Could you check a few things on this model? Use its own coordinates, in mm. Coordinates: 2 decimals unless noted, no trailing zeros. Write each loop counter-clockwise with the first axis right and the second up, starting at its lowest first coordinate (ties: lowest second). Pieces come first, ordered by that corner, then holes. Notation, with made-up numbers: (61, 27) - (117, 27) arc R29 ccw to (117, 51) - close; hole circle Ø11 at (22.25, 39.5). An arc over 180 degrees is marked (long way). Answer as a JSON object with one key per item and string values. Group by question number.
1) Will these pins go through, and if not, where does the flat tip stop? pin 1 Ø7.5 at (x, y) = (56, 6.5) entering from +Z; pin 2 Ø5.5 at (x, y) = (5, 5) entering from +Z.
2) If we section it at A-A (y = 5): Write out the boundary of the cut face in (x, z).
3) Please list where these lines run through material, in increasing order: line 1 along Y through (x, z) = (55, 0.55); line 2 along Y through (x, z) = (5, 1.9); line 3 along Y through (x, z) = (54, 3.4).
4) If we section it at D-D (z = 2.7): Write out the boundary of the cut face in (x, y).
5) If we section it at C-C (y = 55): Write out the boundary of the cut face in (x, z).
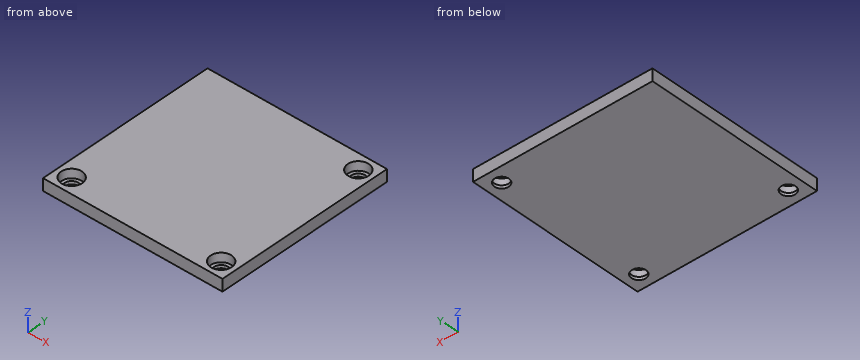
```python
from build123d import *

# Parameters (mm, degrees)
CYLINDER005_R     = 3.5
CYLINDER005_DEPTH = 3
CYLINDER004_R     = 2.4
CYLINDER004_DEPTH = 10
CYLINDER007_R     = 3.5
CYLINDER007_DEPTH = 3
CYLINDER006_R     = 2.4
CYLINDER006_DEPTH = 10
CYLINDER009_R     = 3.5
CYLINDER009_DEPTH = 3
CYLINDER008_R     = 2.4
CYLINDER008_DEPTH = 10
BOX001_W          = 60
BOX001_H          = 60
BOX001_DEPTH      = 4


with BuildPart() as cylinder005:
    # Cylinder005 → Cylinder005 (new body)
    with BuildSketch(Plane.XY.offset(1)):
        Circle(CYLINDER005_R)
    extrude(amount=CYLINDER005_DEPTH)


with BuildPart() as fusion004:
    # Cylinder004 → Cylinder004 (new body)
    with BuildSketch(Plane.XY):
        Circle(CYLINDER004_R)
    extrude(amount=CYLINDER004_DEPTH)

    # Fusion004: union Cylinder005
    add(cylinder005.part)


with BuildPart() as fusion004_1:
    # Fusion004 placement: moved
    add(fusion004.part.moved(Location((5, 5, 0))))


with BuildPart() as cylinder007:
    # Cylinder007 → Cylinder007 (new body)
    with BuildSketch(Plane.XY.offset(1)):
        Circle(CYLINDER007_R)
    extrude(amount=CYLINDER007_DEPTH)


with BuildPart() as fusion005:
    # Cylinder006 → Cylinder006 (new body)
    with BuildSketch(Plane.XY):
        Circle(CYLINDER006_R)
    extrude(amount=CYLINDER006_DEPTH)

    # Fusion005: union Cylinder007
    add(cylinder007.part)


with BuildPart() as fusion005_1:
    # Fusion005 placement: moved
    add(fusion005.part.moved(Location((55, 5, 0))))


with BuildPart() as cylinder009:
    # Cylinder009 → Cylinder009 (new body)
    with BuildSketch(Plane.XY.offset(1)):
        Circle(CYLINDER009_R)
    extrude(amount=CYLINDER009_DEPTH)


with BuildPart() as compound001:
    # Cylinder008 → Cylinder008 (new body)
    with BuildSketch(Plane.XY):
        Circle(CYLINDER008_R)
    extrude(amount=CYLINDER008_DEPTH)

    # Fusion006: union Cylinder009
    add(cylinder009.part)


with BuildPart() as compound001_1:
    # Fusion006 placement: moved
    add(compound001.part.moved(Location((55, 55, 0))))

    # Compound001: union Fusion004, Fusion005
    add(fusion004_1.part)
    add(fusion005_1.part)


with BuildPart() as obj1:
    # Box001 → Box001 (new body)
    with BuildSketch(Plane.XY):
        with Locations((30, 30)):
            Rectangle(BOX001_W, BOX001_H)
    extrude(amount=BOX001_DEPTH)

    # Cut002: cut Compound001
    add(compound001_1.part, mode=Mode.SUBTRACT)


solid = obj1.part
```
Here are the results:
{
 "1": {"pin 1": "stops at z = 4", "pin 2": "stops at z = 1"},
 "2": {"outline": "(0, 0) - (2.6, 0) - (2.6, 1) - (1.5, 1) - (1.5, 4) - (0, 4) - close; (7.4, 0) - (52.6, 0) - (52.6, 1) - (51.5, 1) - (51.5, 4) - (8.5, 4) - (8.5, 1) - (7.4, 1) - close; (57.4, 0) - (60, 0) - (60, 4) - (58.5, 4) - (58.5, 1) - (57.4, 1) - close"},
 "3": {"line 1": "y = 0 to 2.6, 7.4 to 52.6, 57.4 to 60", "line 2": "y = 0 to 1.5, 8.5 to 60", "line 3": "y = 0 to 1.65, 8.35 to 51.65, 58.35 to 60"},
 "4": {"outline": "(0, 0) - (60, 0) - (60, 60) - (0, 60) - close; hole circle Ø7 at (5, 5); hole circle Ø7 at (55, 5); hole circle Ø7 at (55, 55)"},
 "5": {"outline": "(0, 0) - (52.6, 0) - (52.6, 1) - (51.5, 1) - (51.5, 4) - (0, 4) - close; (57.4, 0) - (60, 0) - (60, 4) - (58.5, 4) - (58.5, 1) - (57.4, 1) - close"}
}
